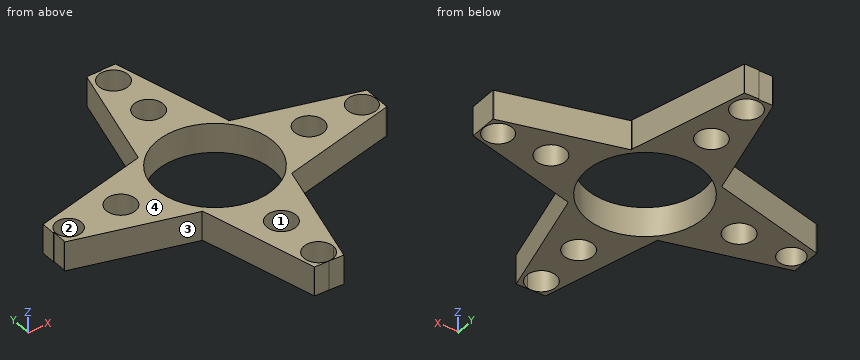
from build123d import *

# Parameters (mm, degrees)
F0_R     = 3.075923
F0_R_2   = 3.497253
F0_R_3   = 3.40731
F0_R_4   = 13.899926
F0_R_5   = 3.497252
F1_DEPTH = 7


with BuildPart() as f1:
    # F0 (on Top) → F1 (new body)
    with BuildSketch(Plane.XY):
        with BuildLine():
            ThreePointArc((0.996115, -38.345504), (2.803066, -37.084421), (3.497242, -34.993124))
            ThreePointArc((3.497242, -34.993124), (-2.803066, -32.901827), (0.996115, -38.345504))
        make_face()
        Polygon((0, -38.515605), (3.472779, -38.609888), (10.659512, -10.923896), (10.713998, -10.713998), (38.329154, -3.497253), (38.515605, -3.497253), (38.515605, 0), (38.515605, 3.317366), (38.345504, 3.317366), (10.659512, 10.5041), (10.713998, 10.713998), (3.497253, 38.329154), (3.497253, 38.515605), (0, 38.515605), (0.089943, 38.345504), (-3.317366, 38.345504), (-3.58175, 38.190092), (-10.713998, 10.713998), (-38.329154, 3.497253), (-38.515605, 3.497253), (-38.515605, 0), (-38.345504, 0.089943), (-38.345504, -3.317366), (-38.454475, -3.737162), (-10.768483, -10.923896), (-10.713998, -10.713998), (-3.497253, -38.329154), (-3.497253, -38.515605), align=None)
        with Locations((-35.088168, -0.30512)):
            Circle(F0_R, mode=Mode.SUBTRACT)
        with BuildLine():
            ThreePointArc((0.996115, -38.345504), (-2.803066, -32.901827), (3.497242, -34.993124))
            ThreePointArc((3.497242, -34.993124), (2.803066, -37.084421), (0.996115, -38.345504))
        make_face(mode=Mode.SUBTRACT)
        with Locations((0, -22.420802)):
            Circle(F0_R_2, mode=Mode.SUBTRACT)
        with Locations((34.938195, -0.089943)):
            Circle(F0_R_3, mode=Mode.SUBTRACT)
        with Locations((-22.420802, 0)):
            Circle(F0_R_2, mode=Mode.SUBTRACT)
        Circle(F0_R_4, mode=Mode.SUBTRACT)
        with Locations((22.420802, 0)):
            Circle(F0_R_2, mode=Mode.SUBTRACT)
        with Locations((0, 22.420802)):
            Circle(F0_R_2, mode=Mode.SUBTRACT)
        with Locations((0, 34.286165)):
            Circle(F0_R_5, mode=Mode.SUBTRACT)
    extrude(amount=F1_DEPTH)


solid = f1.part
Design review of the part built by this model. Coordinates are the model's own, in mm. Face numbers are marked on the shaded views. Round coordinates to 2 decimals unless told otherwise and drop trailing zeros. Write each loop counter-clockwise with the first axis right and the second up, starting at its lowest first coordinate (ties: lowest second). Pieces come first, ordered by that corner, then holes.
Item 1: For pin 1 Ø1 at (x, z) = (3.5, 6) entering from -Y; pin 2 Ø1 at (x, z) = (-1.5, 3.5) entering from +Y; pin 3 Ø4 at (y, z) = (-23, 2) entering from +X; pin 4 Ø1.5 at (y, z) = (-15, 2) entering from -X, all flat-tipped, find the tip position at first contact; note any pin that passes through.
Item 2: Draft analysis for pull direction Y (two halves, no side actions). For the marked faces 1, 2, 3 and 4, state which applies: released by +Y, released by -Y, zero draft, split by the parting line, or undercut.
Item 3: Consider section C-C on z = 5.5. Count the separate pieces of the cut face and the enclosed holes in it, and give its area (3 significant figures).
Item 4: Consider section A-A on y = 21.5. Give the boundary of the cut face in (x, z), and give its area (3 significant figures).
Item 5: Wall thickness on L1, parallel to Y at x = 21.5, z = 1.5; L2, parallel to Y at x = 2.5, z = 0.5; L3, parallel to X at y = 1.5, z = 6.5: over which ranges is each line inside the solid? List them lowest first.
Item 6: Consider section B-B on y = 1. Give the boundary of the cut face in (x, z).
Check values:
1. pin 1: stops at y = -38.61
1. pin 2: stops at y = 38.35
1. pin 3: stops at x = 8.04
1. pin 4: stops at x = -9.79
2. face 1: undercut
2. face 2: undercut
2. face 3: released by -Y
2. face 4: zero draft
3. separate pieces: 1
3. enclosed holes: 9
3. area: 1,130 mm2
4. outline: (-7.91, 0) - (-3.37, 0) - (-3.37, 7) - (-7.91, 7) - close; (3.37, 0) - (7.9, 0) - (7.9, 7) - (3.37, 7) - close
4. area: 63.4 mm2
5. L1: y = -7.9 to -3.37, 3.37 to 7.69
5. L2: y = -38.58 to -37.44, -32.55 to -24.87, -19.98 to -13.67, 13.67 to 19.98, 24.87 to 31.84, 36.73 to 38.52
5. L3: x = -38.52 to -37.58, -32.6 to -25.58, -19.26 to -13.82, 13.82 to 19.26, 25.58 to 31.92, 37.95 to 38.52
6. outline: (-38.52, 0) - (-37.87, 0) - (-37.87, 7) - (-38.52, 7) - close; (-32.3, 0) - (-25.77, 0) - (-25.77, 7) - (-32.3, 7) - close; (-19.07, 0) - (-13.86, 0) - (-13.86, 7) - (-19.07, 7) - close; (13.86, 0) - (19.07, 0) - (19.07, 7) - (13.86, 7) - close; (25.77, 0) - (31.71, 0) - (31.71, 7) - (25.77, 7) - close; (38.17, 0) - (38.52, 0) - (38.52, 7) - (38.17, 7) - close
